Geometry check sheet. Reference: the model listing, model coordinates, mm. A direction names the side the tool comes from. Round coordinates to 2 decimals unless told otherwise and drop trailing zeros. Order: outer loops, then holes, each group sorted by start corner. A loop starts at its lowest first (then second) coordinate and runs counter-clockwise, first axis right, second up. Notation, with made-up numbers: (14, -28.75) - (46, -28.75) arc R20 ccw to (46, -13.75) - close; hole circle Ø6 at (51, 0.5). An arc over 180 degrees is marked (long way). One line per question, with ' | ' between items. Start each with the question number.
Q1. Sectioned sample at B-B, the plane z = 30. Enter the section's corners in (x, y), then the cut area to 3 significant figures.
Q2. Tool access check on faces 1 (the face through (0.021, -3.042, 37.385)), 2 (the face through (-6, -30, 42.5)), 3 (the face through (2.36, -31.1, 51.37)). Record the directions out of +Z, -Z, +X, -X, +Y, -Y that give a thin tool (end or side, any length) a straight path to the whole face; none if there is none.
Q3. Sectioned sample at C-C, the plane x = 10. Enter the section's corners in (y, z), then the cut area to 3 significant figures.
Q4. Sectioned sample at D-D, the plane y = 6.5. Enter the section's corners in (x, z), then the cut area to 3 significant figures.
Q5. Mould release check, pull along Y, two halves, no side actions. Record for faces 4 (the face through (-9, -28, 30)), 5 (the face through (0, -35, 30)), 6 (the face through (0.021, 15.905, 37.336)), 7 (the face through (10.07, -33.52, 51.5)): +Y half, -Y half, draft (parallel to the pull), parting line (faces both ways), or undercut.
Q6. Material ranges on line 1 along X through (y, z) = (-33, 50); line 2 along Y through (x, z) = (-10.5, 56); line 3 along X through (y, z) = (15.5, 42), recorded low to high.
Q7. Sectioned sample at A-A, the plane y = 19.05. Enter the section's corners in (x, z), then the cut area to 3 significant figures.
Q8. Gauge pin test, flat ends, axial feed: P1, Ø6, axis at x = -8, z = 8, coming from the +Y side; P2, Ø2, axis at y = -0.5, z = 51, coming from the +X side; P3, Ø2.5, axis at x = 10, z = 10, coming from the +Y side; P4, Ø9, axis at y = 6.5, z = 30, coming from the -X side. Record the tip position at first contact, or that the pin passes through.
```python
from build123d import *

# Parameters (mm, degrees)
SKETCH_1_W               = 3
SKETCH_1_H               = 70
EXTRUDE_1_DEPTH          = 60
SKETCH_2_W               = 60
SKETCH_2_H               = 3
EXTRUDE_2_DEPTH          = 15
FILLET_2_R               = 10
CUT_EXTRUDE_1_REACH      = 73.757
SKETCH_3_R               = 1.65
SKETCH_3_R_2             = 4
SKETCH_5_R               = 1.5
CUT_EXTRUDE_4_DEPTH      = 3
FILLET_3_R               = 10
MIRROR_3_COPY_1_SKETCH_R = 1.5
MIRROR_3_COPY_1_DEPTH    = 3
MIRROR_3_COPY_2_SKETCH_R = 1.5
MIRROR_3_COPY_2_DEPTH    = 3
SKETCH_7_R               = 1.65
CUT_EXTRUDE_5_DEPTH      = 10
EXTRUDE_3_DEPTH          = 12.5
FILLET_4_R               = 3


with BuildPart() as part:
    # 草图1 → 凸台-拉伸1 (new body)
    with BuildSketch(Plane.XY):
        Rectangle(SKETCH_1_W, SKETCH_1_H)
    extrude(amount=EXTRUDE_1_DEPTH)

    # 草图2 → 凸台-拉伸2 (add)
    with BuildSketch(Plane.ZY.offset(1.5)):
        with Locations((30, -33.5)):
            Rectangle(SKETCH_2_W, SKETCH_2_H)
    extrude_2 = extrude(amount=EXTRUDE_2_DEPTH)

    # 镜向1: 凸台-拉伸2 across plane
    add(extrude_2.mirror(Plane(origin=(0, 0, 0), x_dir=(0, 0, 1), z_dir=(1, 0, 0))))

    # 圆角2
    fillet_2_edges = [part.edges().sort_by_distance(p)[0] for p in [
        (0, 35, 0),
        (0, 35, 60),
    ]]
    fillet(fillet_2_edges, radius=FILLET_2_R)

    # 草图3 → 切除-拉伸1 (cut, up to next)
    with BuildSketch(Plane(origin=(1.5, 0, 0), x_dir=(0, 0, -1), z_dir=(1, 0, 0)), mode=Mode.PRIVATE) as cut_extrude_1_sk1:
        with Locations((-38.909545443, -2.409545443)):
            Circle(SKETCH_3_R)
    cut_extrude_1_tool1 = extrude(cut_extrude_1_sk1.sketch, amount=-CUT_EXTRUDE_1_REACH, mode=Mode.PRIVATE) & part.part
    # 草图3 → 切除-拉伸1 (cut, up to next)
    with BuildSketch(Plane(origin=(1.5, 0, 0), x_dir=(0, 0, -1), z_dir=(1, 0, 0)), mode=Mode.PRIVATE) as cut_extrude_1_sk2:
        with Locations((-21.090454557, -2.409545443)):
            Circle(SKETCH_3_R)
    cut_extrude_1_tool2 = extrude(cut_extrude_1_sk2.sketch, amount=-CUT_EXTRUDE_1_REACH, mode=Mode.PRIVATE) & part.part
    # 草图3 → 切除-拉伸1 (cut, up to next)
    with BuildSketch(Plane(origin=(1.5, 0, 0), x_dir=(0, 0, -1), z_dir=(1, 0, 0)), mode=Mode.PRIVATE) as cut_extrude_1_sk3:
        with Locations((-30, 6.5)):
            Circle(SKETCH_3_R_2)
    cut_extrude_1_tool3 = extrude(cut_extrude_1_sk3.sketch, amount=-CUT_EXTRUDE_1_REACH, mode=Mode.PRIVATE) & part.part
    # 草图3 → 切除-拉伸1 (cut, up to next)
    with BuildSketch(Plane(origin=(1.5, 0, 0), x_dir=(0, 0, -1), z_dir=(1, 0, 0)), mode=Mode.PRIVATE) as cut_extrude_1_sk4:
        with Locations((-38.909545443, 15.409545443)):
            Circle(SKETCH_3_R)
    cut_extrude_1_tool4 = extrude(cut_extrude_1_sk4.sketch, amount=-CUT_EXTRUDE_1_REACH, mode=Mode.PRIVATE) & part.part
    # 草图3 → 切除-拉伸1 (cut, up to next)
    with BuildSketch(Plane(origin=(1.5, 0, 0), x_dir=(0, 0, -1), z_dir=(1, 0, 0)), mode=Mode.PRIVATE) as cut_extrude_1_sk5:
        with Locations((-21.090454557, 15.409545443)):
            Circle(SKETCH_3_R)
    cut_extrude_1_tool5 = extrude(cut_extrude_1_sk5.sketch, amount=-CUT_EXTRUDE_1_REACH, mode=Mode.PRIVATE) & part.part
    add(cut_extrude_1_tool1.solids().sort_by_distance((1.5, -2.409545, 38.909545))[0], mode=Mode.SUBTRACT)
    add(cut_extrude_1_tool2.solids().sort_by_distance((1.5, -2.409545, 21.090455))[0], mode=Mode.SUBTRACT)
    add(cut_extrude_1_tool3.solids().sort_by_distance((1.5, 6.5, 30))[0], mode=Mode.SUBTRACT)
    add(cut_extrude_1_tool4.solids().sort_by_distance((1.5, 15.409545, 38.909545))[0], mode=Mode.SUBTRACT)
    add(cut_extrude_1_tool5.solids().sort_by_distance((1.5, 15.409545, 21.090455))[0], mode=Mode.SUBTRACT)

    # 草图5 → 切除-拉伸4 (cut)
    with BuildSketch(Plane(origin=(0, -35, 0), x_dir=(1, 0, 0), z_dir=(0, 1, 0))):
        with Locations(Location((10, -10, 0), (0, 0, 270))):
            Circle(SKETCH_5_R)
    cut_extrude_4 = extrude(amount=CUT_EXTRUDE_4_DEPTH, mode=Mode.SUBTRACT)

    # 圆角3
    fillet_3_edges = [part.edges().sort_by_distance(p)[0] for p in [
        (-16.5, -33.5, 0),
        (-16.5, -33.5, 60),
        (16.5, -33.5, 60),
        (16.5, -33.5, 0),
    ]]
    fillet(fillet_3_edges, radius=FILLET_3_R)

    # 镜向2: 切除-拉伸4 across plane
    add(cut_extrude_4.mirror(Plane(origin=(0, 0, 0), x_dir=(0, 0, 1), z_dir=(1, 0, 0))), mode=Mode.SUBTRACT)

    # 镜向2 at the second plane: 切除-拉伸4 across plane
    add(cut_extrude_4.mirror(Plane.ZX), mode=Mode.SUBTRACT)

    # 镜向3: 切除-拉伸4 across plane
    add(cut_extrude_4.mirror(Plane.XY.offset(30)), mode=Mode.SUBTRACT)

    # 镜向3 copy 1 sketch → 镜向3 copy 1 (cut)
    with BuildSketch(Plane(origin=(0, -35, 60), x_dir=(-1, 0, 0), z_dir=(0, 1, 0))):
        with Locations(Location((10, -10, 0), (0, 0, 270))):
            Circle(MIRROR_3_COPY_1_SKETCH_R)
    extrude(amount=MIRROR_3_COPY_1_DEPTH, mode=Mode.SUBTRACT)

    # 镜向3 copy 2 sketch → 镜向3 copy 2 (cut)
    with BuildSketch(Plane(origin=(0, 35, 60), x_dir=(1, 0, 0), z_dir=(0, -1, 0))):
        with Locations(Location((10, -10, 0), (0, 0, 270))):
            Circle(MIRROR_3_COPY_2_SKETCH_R)
    extrude(amount=MIRROR_3_COPY_2_DEPTH, mode=Mode.SUBTRACT)

    # 草图7 → 切除-拉伸5 (cut)
    with BuildSketch(Plane.ZY.offset(1.5)):
        with Locations((30, 19.05)):
            Circle(SKETCH_7_R)
        with Locations((30, -6.05)):
            Circle(SKETCH_7_R)
    extrude(amount=-CUT_EXTRUDE_5_DEPTH, mode=Mode.SUBTRACT)

    # 草图8 → 凸台-拉伸3 (add, symmetric)
    with BuildSketch(Plane.XY.offset(30)):
        Polygon((1.5, -24), (16.5, -32), (1.5, -32), align=None)
    extrude_3 = extrude(amount=EXTRUDE_3_DEPTH, both=True)

    # 镜向4: 凸台-拉伸3 across plane
    add(extrude_3.mirror(Plane(origin=(0, 0, 0), x_dir=(0, 0, 1), z_dir=(1, 0, 0))))

    # 圆角4
    fillet_4_edges = [part.edges().sort_by_distance(p)[0] for p in [
        (1.5, -32, 51.25),
        (-1.5, -32, 51.25),
        (-1.5, -32, 8.75),
        (1.5, -32, 8.75),
    ]]
    fillet(fillet_4_edges, radius=FILLET_4_R)


solid = part.part
```
Determined:
1) outline: (-16.5, -35) - (16.5, -35) - (16.5, -32) - (1.5, -24) - (1.5, -7.7) - (-1.5, -7.7) - (-1.5, -24) - (-16.5, -32) - close; (-1.5, -4.4) - (1.5, -4.4) - (1.5, 2.5) - (-1.5, 2.5) - close; (-1.5, 10.5) - (1.5, 10.5) - (1.5, 17.4) - (-1.5, 17.4) - close; (-1.5, 20.7) - (1.5, 20.7) - (1.5, 35) - (-1.5, 35) - close | area: 376 mm2
2) face 1: +X, -X | face 2: +Z, -X, +Y | face 3: +Z, +X, +Y
3) outline: (-35, 0.63) - (-32, 0.63) - (-32, 8.5) - (-35, 8.5) - close; (-35, 11.5) - (-32, 11.5) - (-32, 17.5) - (-28.53, 17.5) - (-28.53, 42.5) - (-32, 42.5) - (-32, 48.5) - (-35, 48.5) - close; (-35, 51.5) - (-32, 51.5) - (-32, 59.37) - (-35, 59.37) - close | area: 245 mm2
4) outline: (-1.5, 0) - (1.5, 0) - (1.5, 26) - (-1.5, 26) - close; (-1.5, 34) - (1.5, 34) - (1.5, 60) - (-1.5, 60) - close | area: 156 mm2
5) face 4: +Y half | face 5: -Y half | face 6: undercut | face 7: draft
6) line 1: x = -16.5 to -11.5, -8.5 to 8.5, 11.5 to 16.5 | line 2: y = -35 to -32 | line 3: x = -1.5 to 1.5
7) outline: (-1.5, 0) - (1.5, 0) - (1.5, 28.35) - (-1.5, 28.35) - close; (-1.5, 31.65) - (1.5, 31.65) - (1.5, 60) - (-1.5, 60) - close | area: 170 mm2
8) P1: stops at y = -32 | P2: stops at x = 1.5 | P3: passes through | P4: stops at x = -1.5
